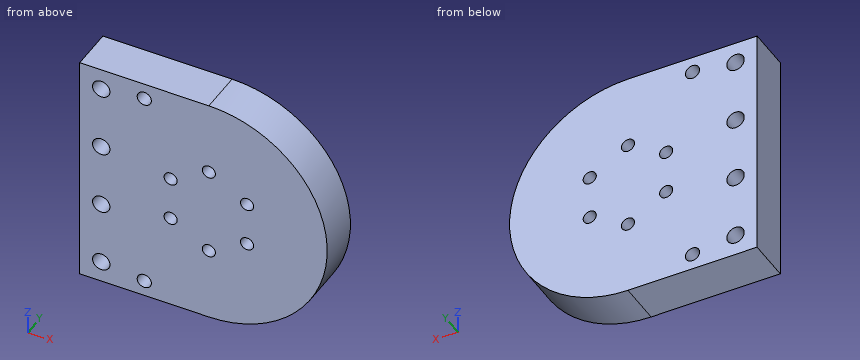
```python
from build123d import *

# Parameters (mm, degrees)
SKETCH_1_R      = 1.65
SKETCH_1_R_2    = 1.525
SKETCH_1_W      = 10
SKETCH_1_H      = 55
SKETCH_1_R_3    = 2.025
EXTRUDE_1_DEPTH = 10


with BuildPart() as part:
    # 草图1 → 凸台-拉伸1 (new body)
    # profile 1 of 2: a face of its own
    with BuildSketch(Plane(origin=(0, 0, 0), x_dir=(1, 0, 0), z_dir=(0, 1, 0))):
        with BuildLine():
            ThreePointArc((0, -27.5), (27.5, 0), (0, 27.5))
            Line((0, 27.5), (-20, 27.5))
            Line((-20, 27.5), (-20, -27.5))
            Line((-20, -27.5), (0, -27.5))
        make_face()
        with Locations(Location((-15, -23.75, 0), (0, 0, 270))):
            Circle(SKETCH_1_R, mode=Mode.SUBTRACT)
        with Locations(Location((-8.876760389, -5.125, 0), (0, 0, 270))):
            Circle(SKETCH_1_R_2, mode=Mode.SUBTRACT)
        with Locations(Location((0, -10.25, 0), (0, 0, 270))):
            Circle(SKETCH_1_R_2, mode=Mode.SUBTRACT)
        with Locations(Location((8.876760389, -5.125, 0), (0, 0, 270))):
            Circle(SKETCH_1_R_2, mode=Mode.SUBTRACT)
        with Locations(Location((-8.876760389, 5.125, 0), (0, 0, 270))):
            Circle(SKETCH_1_R_2, mode=Mode.SUBTRACT)
        with Locations(Location((-15, 23.75, 0), (0, 0, 270))):
            Circle(SKETCH_1_R, mode=Mode.SUBTRACT)
        with Locations(Location((8.876760389, 5.125, 0), (0, 0, 270))):
            Circle(SKETCH_1_R_2, mode=Mode.SUBTRACT)
        with Locations(Location((0, 10.25, 0), (0, 0, 270))):
            Circle(SKETCH_1_R_2, mode=Mode.SUBTRACT)
    # profile 2 of 2: a face of its own
    with BuildSketch(Plane(origin=(0, 0, 0), x_dir=(1, 0, 0), z_dir=(0, 1, 0))):
        with Locations((-25, 0)):
            Rectangle(SKETCH_1_W, SKETCH_1_H)
        with Locations(Location((-25, -22.5, 0), (0, 0, 270))):
            Circle(SKETCH_1_R_3, mode=Mode.SUBTRACT)
        with Locations(Location((-25, -7.5, 0), (0, 0, 270))):
            Circle(SKETCH_1_R_3, mode=Mode.SUBTRACT)
        with Locations(Location((-25, 7.5, 0), (0, 0, 270))):
            Circle(SKETCH_1_R_3, mode=Mode.SUBTRACT)
        with Locations(Location((-25, 22.5, 0), (0, 0, 270))):
            Circle(SKETCH_1_R_3, mode=Mode.SUBTRACT)
    extrude(amount=EXTRUDE_1_DEPTH)


solid = part.part
```
Here's how the part is built. I have some questions about the finished solid (model axes, mm). Give positions to 0.01 mm unless a question says otherwise; leave off trailing zeros. Write each loop counter-clockwise with the first axis right and the second up, starting at its lowest first coordinate (ties: lowest second). Pieces come first, ordered by that corner, then holes.
(1) Imagine slicing it at B-B, the plane z = -7.5. Write out the boundary of the cut face in (x, y) (3 decimals), and give its area (3 significant figures).
Output values:
outline: (-30, 0) - (-27.025, 0) - (-27.025, 10) - (-30, 10) - close; (-22.975, 0) - (26.458, 0) - (26.458, 10) - (-22.975, 10) - close
area: 524 mm2
(2) Imagine slicing it at A-A, the plane x = -25. Write out the boundary of the cut face in (y, z) (3 decimals), and give its area (3 significant figures).
Output values:
outline: (0, -27.5) - (10, -27.5) - (10, -24.525) - (0, -24.525) - close; (0, -20.475) - (10, -20.475) - (10, -9.525) - (0, -9.525) - close; (0, -5.475) - (10, -5.475) - (10, 5.475) - (0, 5.475) - close; (0, 9.525) - (10, 9.525) - (10, 20.475) - (0, 20.475) - close; (0, 24.525) - (10, 24.525) - (10, 27.5) - (0, 27.5) - close
area: 388 mm2
(3) Will these pins go through, and if not, where does the flat tip stop? pin 1 (3.5 mm diameter, centred on x = -8.88, z = -5.12, fed in from -Y); pin 2 (5 mm diameter, centred on y = 6.5, z = -16, fed in from +X); pin 3 (1.5 mm diameter, centred on y = 8, z = -9.5, fed in from +X).
Output values:
pin 1: stops at y = 0
pin 2: stops at x = 23.96
pin 3: stops at x = 26.07
(4) If I drill on L1, parallel to X at y = 8.5, z = 9; L2, parallel to Z at x = -14, y = 7.75; L3, parallel to X at y = 1, z = 23, over which ranges is the centre line in solid material (lowest first)?
Output values:
L1: x = -30 to -26.36, -23.64 to -0.87, 0.87 to 25.99
L2: z = -27.5 to -25.06, -22.44 to 22.44, 25.06 to 27.5
L3: x = -30 to -26.96, -23.04 to -16.47, -13.53 to 15.07
(5) Imagine slicing it at D-D, the plane x = 14.5. Write out the boundary of the cut face in (y, z), and give its area (3 significant figures).
Output values:
outline: (0, -23.37) - (10, -23.37) - (10, 23.37) - (0, 23.37) - close
area: 467 mm2
(6) Imagine slicing it at C-C, the plane y = 8.5. Count the separate pieces of the cut face and the enclosed holes in it, and give its area (3 significant figures).
Output values:
separate pieces: 1
enclosed holes: 12
area: 2,730 mm2
